Could you check a few things on this model? Use its own coordinates, in mm. A direction names the side the tool comes from. Coordinates: 2 decimals unless noted, no trailing zeros. Order: outer loops, then holes, each group sorted by start corner. A loop starts at its lowest first (then second) coordinate and runs counter-clockwise, first axis right, second up. Notation, with made-up numbers: (41, 88) -> (69, 88) arc R23 cw to (69, 101) -> close; hole circle Ø2 at (80, 21.25). An arc over 180 degrees is marked (long way). Put each result on its own line as item: value. Start each with the question number.
Q1. We'd pull the mould along Z, two halves only. Please class faces 5 (the face through (0, 39, 22)), 6 (the face through (38, 42.107, 7)), 7 (the face through (-0.388, 45.025, 17.465)): +Z half, -Z half, draft (parallel to the pull), parting line (faces both ways), or undercut.
Q2. Please list where these lines run through material, in increasing order: line 1 along X through (y, z) = (44.8, 18); line 2 along X through (y, z) = (10, -12); line 3 along X through (y, z) = (45.55, -18).
Q3. For faces 1 (the face through (42, 19, -17)), 2 (the face through (25.165, 45.025, 0.28)), 3 (the face through (29.25, 35.09, -0.43)), 4 (the face through (42.7, 45, 8)), which set-ups out of +Z, -Z, +X, -X, +Y, -Y let a thin tool reach every point of the face, with its end or its side?
Q4. If we section it at A-A (z = 10): Please give me the cut outline in (x, y), and give its area (3 significant figures).
Q5. If we section it at D-D (y = 15): Please give me the cut outline in (x, z), and give its area (3 significant figures).
Q6. If we section it at C-C (y = 28.5): Count the separate pieces of the cut face and the enclosed holes in it, and give its area (3 significant figures).
Q7. Will these pins go through, and if not, where does the flat tip stop? pin 1 (0.5 mm diameter, centred on y = 22, z = -5.5, fed in from -X); pin 2 (1.2 mm diameter, centred on x = 47, z = -17, fed in from -Y); pin 3 (5 mm diameter, centred on y = 24.5, z = 10.5, fed in from -X).
Q8. If we section it at B-B (x = 10.5): Please give me the cut outline in (y, z).
from build123d import *

# Parameters (mm, degrees)
SKETCH1_W           = 65.4
SKETCH1_H           = 60
SKETCH1_W_2         = 45.4
SKETCH1_H_2         = 30
BOSS_EXTRUDE1_DEPTH = 40
SKETCH2_R           = 8
CUT_EXTRUDE1_DEPTH  = 66.4
SKETCH3_W           = 45.4
SKETCH3_H           = 52
CUT_EXTRUDE2_DEPTH  = 37
CHAMFER1_SIZE       = 5
CHAMFER1_SIZE2      = 2.886751346
SKETCH7_W           = 65.4
SKETCH7_H           = 5
CUT_EXTRUDE5_DEPTH  = 41
CHAMFER2_SIZE       = 3
CHAMFER2_SIZE2      = 2.701212133
SKETCH8_W           = 65.4
SKETCH8_H           = 55
SKETCH8_W_2         = 45.4
SKETCH8_H_2         = 30
BOSS_EXTRUDE2_DEPTH = 10
CHAMFER3_SIZE       = 5
CHAMFER3_SIZE2      = 9.813052528
SKETCH10_R          = 11.1
CUT_EXTRUDE8_DEPTH  = 7
SKETCH11_R          = 11.1
CUT_EXTRUDE9_DEPTH  = 7
SKETCH12_W          = 65.4
SKETCH12_H          = 8.2
CUT_EXTRUDE10_DEPTH = 20
SKETCH13_W          = 65.4
SKETCH13_H          = 5
CUT_EXTRUDE11_DEPTH = 3
CHAMFER4_SIZE       = 5
SKETCH20_W          = 50
SKETCH20_H          = 5
BOSS_EXTRUDE5_DEPTH = 10
SKETCH21_W          = 50
SKETCH21_H          = 5
BOSS_EXTRUDE6_DEPTH = 10
CHAMFER5_SIZE       = 5
SKETCH23_R          = 1.6
CUT_EXTRUDE15_DEPTH = 48
SKETCH24_W          = 13.9
SKETCH24_H          = 10
BOSS_EXTRUDE7_DEPTH = 15
SKETCH22_R          = 1.6
CUT_EXTRUDE14_DEPTH = 48.107149008
SKETCH25_R          = 3.5
CUT_EXTRUDE16_DEPTH = 10
SKETCH27_W          = 6
SKETCH27_H          = 10
BOSS_EXTRUDE8_DEPTH = 6.6
CUT_EXTRUDE18_DEPTH = 1.3
SKETCH29_W          = 19.2
SKETCH29_H          = 3.2
CUT_EXTRUDE19_DEPTH = 1.3
SKETCH30_R          = 1.6
CUT_EXTRUDE20_DEPTH = 56
CUT_EXTRUDE21_DEPTH = 3
SKETCH32_R          = 3.15
CUT_EXTRUDE22_DEPTH = 5
SKETCH35_W          = 105.7739029
SKETCH35_H          = 101.810214422
CUT_EXTRUDE23_DEPTH = 5
CHAMFER6_SIZE       = 5
CUT_EXTRUDE25_DEPTH = 43
SKETCH37_R          = 3.5
BOSS_EXTRUDE9_DEPTH = 18.107149


with BuildPart() as part:
    # Sketch1 → Boss-Extrude1 (new body)
    with BuildSketch(Plane(origin=(0, 0, 0), x_dir=(1, 0, 0), z_dir=(0, 1, 0))):
        Rectangle(SKETCH1_W, SKETCH1_H)
        Rectangle(SKETCH1_W_2, SKETCH1_H_2, mode=Mode.SUBTRACT)
    extrude(amount=BOSS_EXTRUDE1_DEPTH)

    # Sketch2 → Cut-Extrude1 (cut, through all)
    with BuildSketch(Plane(origin=(32.7, 0, 0), x_dir=(0, 0, -1), z_dir=(1, 0, 0))):
        with Locations((0, 24)):
            Circle(SKETCH2_R)
    extrude(amount=-CUT_EXTRUDE1_DEPTH, mode=Mode.SUBTRACT)

    # Sketch3 → Cut-Extrude2 (cut)
    with BuildSketch(Plane.XZ):
        Rectangle(SKETCH3_W, SKETCH3_H)
    extrude(amount=-CUT_EXTRUDE2_DEPTH, mode=Mode.SUBTRACT)

    # Chamfer1
    chamfer1_edges = [part.edges().sort_by_distance(p)[0] for p in [
        (0, 37, -15),
    ]]
    chamfer1_side = [part.faces().sort_by_distance(p)[0] for p in [
        (0, 37, -20.5),
    ]]
    chamfer(chamfer1_edges, length=CHAMFER1_SIZE, length2=CHAMFER1_SIZE2, reference=chamfer1_side[0])

    # Sketch7 → Cut-Extrude5 (cut, through all)
    with BuildSketch(Plane(origin=(0, 40, 0), x_dir=(1, 0, 0), z_dir=(0, 1, 0))):
        with Locations((0, -27.5)):
            Rectangle(SKETCH7_W, SKETCH7_H)
    extrude(amount=-CUT_EXTRUDE5_DEPTH, mode=Mode.SUBTRACT)

    # Chamfer2
    chamfer2_edges = [part.edges().sort_by_distance(p)[0] for p in [
        (0, 37, 15),
    ]]
    chamfer2_side = [part.faces().sort_by_distance(p)[0] for p in [
        (0, 37, 20),
    ]]
    chamfer(chamfer2_edges, length=CHAMFER2_SIZE, length2=CHAMFER2_SIZE2, reference=chamfer2_side[0])

    # Sketch8 → Boss-Extrude2 (add)
    with BuildSketch(Plane(origin=(0, 40, 0), x_dir=(1, 0, 0), z_dir=(0, 1, 0))):
        with Locations((0, 2.5)):
            Rectangle(SKETCH8_W, SKETCH8_H)
        Rectangle(SKETCH8_W_2, SKETCH8_H_2, mode=Mode.SUBTRACT)
    extrude(amount=BOSS_EXTRUDE2_DEPTH)

    # Chamfer3
    chamfer3_edges = [part.edges().sort_by_distance(p)[0] for p in [
        (-22.7, 50, 0),
        (0, 50, 15),
        (22.7, 50, 0),
        (0, 50, -15),
    ]]
    chamfer3_side = [part.faces().sort_by_distance(p)[0] for p in [
        (0, 50, 24.14547323),
    ]]
    chamfer(chamfer3_edges, length=CHAMFER3_SIZE, length2=CHAMFER3_SIZE2, reference=chamfer3_side[0])

    # Sketch10 → Cut-Extrude8 (cut)
    with BuildSketch(Plane(origin=(32.7, 0, 0), x_dir=(0, 0, -1), z_dir=(1, 0, 0))):
        with Locations((0, 24)):
            Circle(SKETCH10_R)
    extrude(amount=-CUT_EXTRUDE8_DEPTH, mode=Mode.SUBTRACT)

    # Sketch11 → Cut-Extrude9 (cut)
    with BuildSketch(Plane.ZY.offset(32.7)):
        with Locations(Location((0, 24, 0), (0, 0, 180))):  # turned: the seam where the file's is
            Circle(SKETCH11_R)
    extrude(amount=-CUT_EXTRUDE9_DEPTH, mode=Mode.SUBTRACT)

    # Sketch12 → Cut-Extrude10 (cut)
    with BuildSketch(Plane.XZ):
        Rectangle(SKETCH12_W, SKETCH12_H)
    extrude(amount=-CUT_EXTRUDE10_DEPTH, mode=Mode.SUBTRACT)

    # Sketch13 → Cut-Extrude11 (cut)
    with BuildSketch(Plane(origin=(0, 50, 0), x_dir=(1, 0, 0), z_dir=(0, 1, 0))):
        with Locations((0, 27.5)):
            Rectangle(SKETCH13_W, SKETCH13_H)
    extrude(amount=-CUT_EXTRUDE11_DEPTH, mode=Mode.SUBTRACT)

    # Chamfer4
    chamfer4_edges = [part.edges().sort_by_distance(p)[0] for p in [
        (-32.7, 23.5, -30),
        (32.7, 23.5, -30),
    ]]
    chamfer(chamfer4_edges, length=CHAMFER4_SIZE)

    # Sketch20 → Boss-Extrude5 (add)
    with BuildSketch(Plane(origin=(32.7, 0, 0), x_dir=(0, 0, -1), z_dir=(1, 0, 0))):
        with Locations((0, 44.607149008)):
            Rectangle(SKETCH20_W, SKETCH20_H)
    extrude(amount=BOSS_EXTRUDE5_DEPTH)

    # Sketch21 → Boss-Extrude6 (add)
    with BuildSketch(Plane.ZY.offset(32.7)):
        with Locations((0, 44.5)):
            Rectangle(SKETCH21_W, SKETCH21_H)
    extrude(amount=BOSS_EXTRUDE6_DEPTH)

    # Chamfer5
    chamfer5_edges = [part.edges().sort_by_distance(p)[0] for p in [
        (42.7, 44.607149008, 25),
        (42.7, 44.607149008, -25),
        (-42.7, 44.5, -25),
        (-42.7, 44.5, 25),
    ]]
    chamfer(chamfer5_edges, length=CHAMFER5_SIZE)

    # Sketch23 → Cut-Extrude15 (cut, through all)
    with BuildSketch(Plane(origin=(0, 47, 0), x_dir=(1, 0, 0), z_dir=(0, 1, 0))):
        with Locations(Location((-37.7, 18, 0), (0, 0, 270))):  # turned: the seam where the file's is
            Circle(SKETCH23_R)
        with Locations(Location((-37.7, -18, 0), (0, 0, 270))):  # turned: the seam where the file's is
            Circle(SKETCH23_R)
    extrude(amount=-CUT_EXTRUDE15_DEPTH, mode=Mode.SUBTRACT)

    # Sketch24 → Boss-Extrude7 (add)
    with BuildSketch(Plane(origin=(32.7, 0, 0), x_dir=(0, 0, -1), z_dir=(1, 0, 0))):
        with Locations((18.05, 24)):
            Rectangle(SKETCH24_W, SKETCH24_H)
    extrude(amount=BOSS_EXTRUDE7_DEPTH)

    # Sketch22 → Cut-Extrude14 (cut, through all)
    with BuildSketch(Plane(origin=(0, 47.107149008, 0), x_dir=(1, 0, 0), z_dir=(0, 1, 0))):
        with Locations(Location((37.7, -18, 0), (0, 0, 270))):  # turned: the seam where the file's is
            Circle(SKETCH22_R)
        with Locations(Location((37.7, 18, 0), (0, 0, 270))):  # turned: the seam where the file's is
            Circle(SKETCH22_R)
    extrude(amount=-CUT_EXTRUDE14_DEPTH, mode=Mode.SUBTRACT)

    # Sketch25 → Cut-Extrude16 (cut)
    with BuildSketch(Plane.XZ.offset(-19)):
        with Locations(Location((37.7, -18, 0), (0, 0, 270))):  # turned: the seam where the file's is
            Circle(SKETCH25_R)
    extrude(amount=-CUT_EXTRUDE16_DEPTH, mode=Mode.SUBTRACT)

    # Sketch27 → Boss-Extrude8 (add)
    with BuildSketch(Plane.XY.offset(-11.1)):
        with Locations((44.7, 24)):
            Rectangle(SKETCH27_W, SKETCH27_H)
    extrude(amount=BOSS_EXTRUDE8_DEPTH)

    # Sketch28 → Cut-Extrude18 (cut)
    with BuildSketch(Plane.XY.offset(-4.5)):
        Polygon((46.25, 21.8), (46.25, 22.4), (47.7, 22.4), (47.7, 25.6), (46.25, 25.6), (46.25, 26.2), (43.15, 26.2), (43.15, 21.8), align=None)
    extrude(amount=-CUT_EXTRUDE18_DEPTH, mode=Mode.SUBTRACT)

    # Sketch29 → Cut-Extrude19 (cut)
    with BuildSketch(Plane(origin=(47.7, 0, 0), x_dir=(0, 0, -1), z_dir=(1, 0, 0))):
        with Locations((15.4, 24)):
            Rectangle(SKETCH29_W, SKETCH29_H)
    extrude(amount=-CUT_EXTRUDE19_DEPTH, mode=Mode.SUBTRACT)

    # Sketch30 → Cut-Extrude20 (cut, through all)
    with BuildSketch(Plane.XY.offset(25)):
        with Locations(Location((-29, 10, 0), (0, 0, 324.340912304))):  # turned: the seam where the file's is
            Circle(SKETCH30_R)
        with Locations(Location((29, 10, 0), (0, 0, 144.340912304))):  # turned: the seam where the file's is
            Circle(SKETCH30_R)
    extrude(amount=-CUT_EXTRUDE20_DEPTH, mode=Mode.SUBTRACT)

    # Sketch31 → Cut-Extrude21 (cut)
    with BuildSketch(Plane.XY.offset(25)):
        Polygon((26.185417438, 11.625), (26.185417438, 8.375), (29, 6.75), (31.814582562, 8.375), (31.814582562, 11.625), (29, 13.25), align=None)
        Polygon((-31.814582562, 11.625), (-31.814582562, 8.375), (-29, 6.75), (-26.185417438, 8.375), (-26.185417438, 11.625), (-29, 13.25), align=None)
    extrude(amount=-CUT_EXTRUDE21_DEPTH, mode=Mode.SUBTRACT)

    # Sketch32 → Cut-Extrude22 (cut)
    with BuildSketch(Plane(origin=(0, 0, -30), x_dir=(-1, 0, 0), z_dir=(0, 0, -1))):
        with Locations((-29, 10)):
            Circle(SKETCH32_R)
        with Locations((29, 10)):
            Circle(SKETCH32_R)
    extrude(amount=-CUT_EXTRUDE22_DEPTH, mode=Mode.SUBTRACT)

    # Sketch35 → Cut-Extrude23 (cut)
    with BuildSketch(Plane.XZ):
        Rectangle(SKETCH35_W, SKETCH35_H)
    extrude(amount=-CUT_EXTRUDE23_DEPTH, mode=Mode.SUBTRACT)

    # Chamfer6
    chamfer6_edges = [part.edges().sort_by_distance(p)[0] for p in [
        (0, 37, 25),
    ]]
    chamfer(chamfer6_edges, length=CHAMFER6_SIZE)

    # Sketch36 → Cut-Extrude25 (cut, through all)
    with BuildSketch(Plane(origin=(0, 47, 0), x_dir=(1, 0, 0), z_dir=(0, 1, 0))):
        Polygon((32.7, 25), (27.7, 30), (-27.7, 30), (-32.7, 25), align=None)
    extrude(amount=-CUT_EXTRUDE25_DEPTH, mode=Mode.SUBTRACT)

    # Sketch37 → Boss-Extrude9 (add)
    with BuildSketch(Plane(origin=(0, 29, 0), x_dir=(1, 0, 0), z_dir=(0, 1, 0))):
        Polygon((32.7, 11.1), (41.7, 11.1), (41.7, 4.5), (47.7, 4.5), (47.7, 25), (32.7, 25), align=None)
        with Locations(Location((37.7, 18, 0), (0, 0, 90))):  # turned: the seam where the file's is
            Circle(SKETCH37_R, mode=Mode.SUBTRACT)
    extrude(amount=BOSS_EXTRUDE9_DEPTH)


solid = part.part
The answers:
1. face 5: +Z half
1. face 6: draft
1. face 7: undercut
2. line 1: -42.7 to -39.3, -36.1 to 36.1, 39.3 to 42.7
2. line 2: -32.7 to -30.6, -27.4 to -22.7, 22.7 to 27.4, 30.6 to 32.7
2. line 3: -42.7 to -39.3, -36.1 to 36.1, 39.3 to 47.7
3. face 1: +Z, -Z, +X, -Y
3. face 2: +Y
3. face 3: none
3. face 4: +Z, +X, +Y, -Y
4. outline: (-42.7, 42) -> (-32.7, 42) -> (-32.7, 28.82) -> (-25.7, 28.82) -> (-25.7, 19.18) -> (-32.7, 19.18) -> (-32.7, 5) -> (-22.7, 5) -> (-22.7, 40.19) -> (-27.7, 50) -> (-32.7, 50) -> (-32.7, 47) -> (-42.7, 47) -> close; (22.7, 5) -> (32.7, 5) -> (32.7, 19.18) -> (25.7, 19.18) -> (25.7, 28.82) -> (32.7, 28.82) -> (32.7, 42.11) -> (42.7, 42.11) -> (42.7, 47.11) -> (32.7, 47.11) -> (32.7, 50) -> (27.7, 50) -> (22.7, 40.19) -> close; hole circle Ø3.2 at (-29, 10); hole circle Ø3.2 at (29, 10)
4. area: 800 mm^2
5. outline: (-32.7, -25) -> (-22.7, -25) -> (-22.7, -4.1) -> (-25.7, -4.1) -> (-25.7, -6.5) -> (-32.7, -6.5) -> close; (-32.7, 6.5) -> (-25.7, 6.5) -> (-25.7, 4.1) -> (-22.7, 4.1) -> (-22.7, 25) -> (-32.7, 25) -> close; (22.7, -25) -> (32.7, -25) -> (32.7, -6.5) -> (25.7, -6.5) -> (25.7, -4.1) -> (22.7, -4.1) -> close; (22.7, 4.1) -> (25.7, 4.1) -> (25.7, 6.5) -> (32.7, 6.5) -> (32.7, 25) -> (22.7, 25) -> close
5. area: 769 mm^2
6. separate pieces: 4
6. enclosed holes: 1
6. area: 846 mm^2
7. pin 1: x = 41.7
7. pin 2: y = 19
7. pin 3: x = -32.7
8. outline: (37, -25) -> (50, -25) -> (50, -20) -> (40.19, -15) -> (39.89, -15) -> (37, -20) -> close; (37, 18) -> (39.7, 15) -> (40.19, 15) -> (50, 20) -> (50, 25) -> (42, 25) -> (37, 20) -> close
